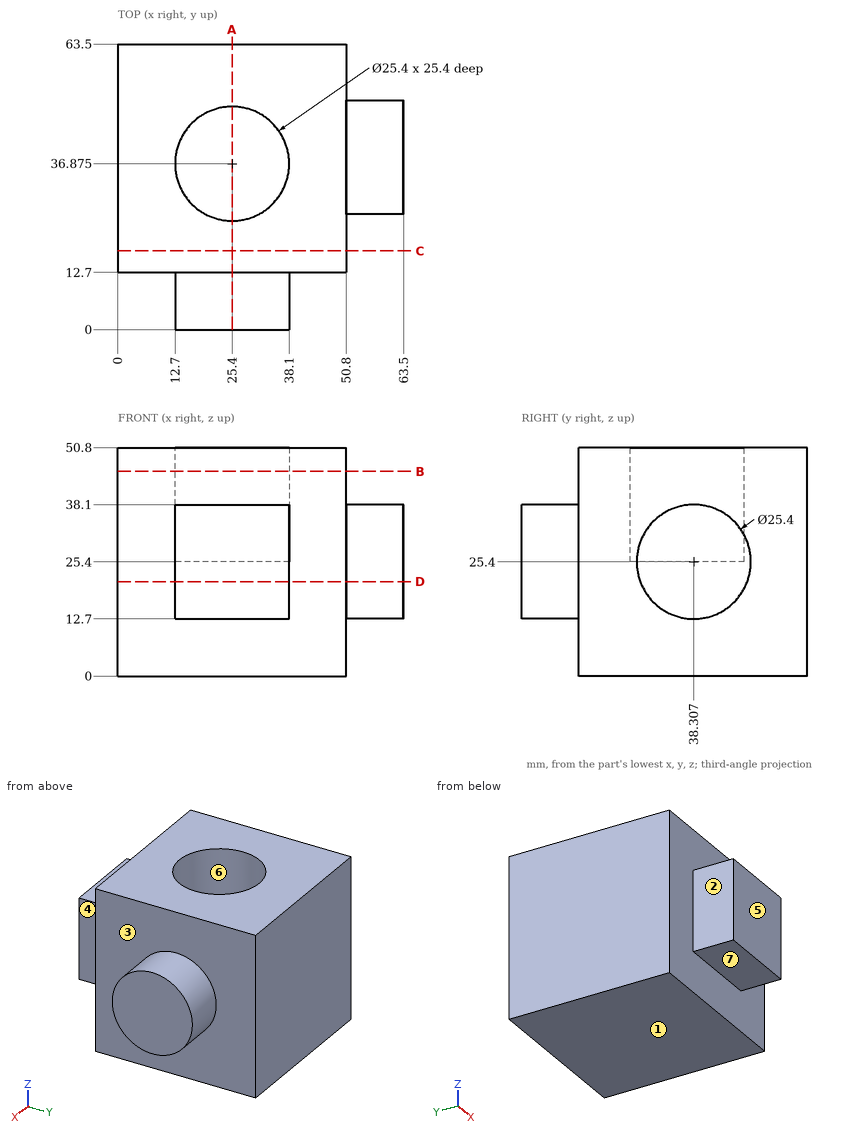
Verification items for this drawing (mm, ordinates from the low corner). A direction names the side the tool comes from. Coordinates: 2 decimals unless noted, no trailing zeros. Loops run counter-clockwise (first coordinate to the right, second up) from the corner with the lowest first, then second, coordinate; pieces in that order, holes last. Notation, with made-up numbers: (11, -8.75) - (45, -8.75) arc R22 cw to (45, 14.25) - close; hole circle Ø11 at (22.25, 87.5). An arc over 180 degrees is marked (long way). One line per item, written item: value. Start each with the question number.
(1) Tool access check on the marked faces 1, 2, 3 and 4. Record the directions out of +Z, -Z, +X, -X, +Y, -Y that give a thin tool (end or side, any length) a straight path to the whole face; none if there is none.
(2) Cross-section at B-B on z = 45.5. Enter the section's corners in (x, y) (1 decimal), plus the area to 3 significant figures.
(3) Depth check by flat-ended pin: P1, Ø4, axis at y = 3.5, z = 20.5, coming from the -X side; P2, Ø10, axis at x = 27.5, y = 3.5, coming from the +Z side; P3, Ø1, axis at x = 39.5, y = 11, coming from the +Z side; P4, Ø3, axis at y = 37.5, z = 10, coming from the +X side. Enter the tip coordinate at first touch or a pass-through.
(4) Mould release check, pull along Y, two halves, no side actions. Record for the marked faces 5, 6 and 7: released by +Y, released by -Y, zero draft, split by the parting line, or undercut.
(5) Cross-section at D-D on z = 21. Enter the section's corners in (x, y).
(6) Cross-section at C-C on y = 17.5. Enter the section's corners in (x, z).
(7) Material ranges on line 1 (Y direction, x = 25, z = 41); line 2 (X direction, y = 5.5, z = 37); line 3 (X direction, y = 57.5, z = 10.5), recorded low to high. Write a range as [from, to].
(8) Cross-section at A-A on x = 25.4. Enter the section's corners in (y, z) (1 decimal), plus the area to 3 significant figures.
Results below:
1. face 1: -Z, +X, -X, +Y, -Y
1. face 2: +Z, -Z, -X, -Y
1. face 3: +X
1. face 4: +Z, -Z, +X, -Y
2. outline: (0, 12.7) - (50.8, 12.7) - (50.8, 63.5) - (0, 63.5) - close; hole circle Ø25.4 at (25.4, 36.9)
2. area: 2,070 mm2
3. P1: stops at x = 12.7
3. P2: stops at z = 38.1
3. P3: passes through
3. P4: stops at x = 50.8
4. face 5: released by -Y
4. face 6: undercut
4. face 7: zero draft
5. outline: (0, 12.7) - (12.7, 12.7) - (12.7, 0) - (38.1, 0) - (38.1, 12.7) - (50.8, 12.7) - (50.8, 26.39) - (63.5, 26.39) - (63.5, 50.22) - (50.8, 50.22) - (50.8, 63.5) - (0, 63.5) - close
6. outline: (0, 0) - (50.8, 0) - (50.8, 50.8) - (0, 50.8) - close
7. line 1: y = [12.7, 24.18], [49.57, 63.5]
7. line 2: x = [12.7, 38.1]
7. line 3: x = [0, 50.8]
8. outline: (0, 12.7) - (12.7, 12.7) - (12.7, 0) - (63.5, 0) - (63.5, 50.8) - (49.6, 50.8) - (49.6, 25.4) - (24.2, 25.4) - (24.2, 50.8) - (12.7, 50.8) - (12.7, 38.1) - (0, 38.1) - close
8. area: 2,260 mm2
